For this review, take the finished solid that the model builds, in its own axes (mm). A direction names the side the tool comes from. Coordinates: 2 decimals unless noted, no trailing zeros. Write each loop counter-clockwise with the first axis right and the second up, starting at its lowest first coordinate (ties: lowest second). Pieces come first, ordered by that corner, then holes.
```python
from build123d import *

# Parameters (mm, degrees)
SKETCH_1_W      = 180
SKETCH_1_H      = 90
EXTRUDE_1_DEPTH = 3
FILLET_1_R      = 1
SKETCH_2_W      = 173
SKETCH_2_H      = 83
EXTRUDE_2_DEPTH = 3
SKETCH_5_R      = 2.695
SKETCH_5_R_2    = 0.895
SKETCH_5_R_3    = 2
SKETCH_5_R_4    = 0.7
SKETCH_5_R_5    = 3.225
SKETCH_5_R_6    = 1.425
EXTRUDE_3_DEPTH = 15.90000066


with BuildPart() as part:
    # 草图1 → 凸台-拉伸1 (new body)
    with BuildSketch(Plane(origin=(0, 0, 0), x_dir=(1, 0, 0), z_dir=(0, 1, 0))):
        Rectangle(SKETCH_1_W, SKETCH_1_H)
    extrude(amount=EXTRUDE_1_DEPTH)

    # 圆角1
    fillet_1_edges = [part.edges().sort_by_distance(p)[0] for p in [
        (0, 0, -45),
        (90, 0, 0),
        (0, 0, 45),
        (-90, 0, 0),
    ]]
    fillet(fillet_1_edges, radius=FILLET_1_R)

    # 草图2 → 凸台-拉伸2 (add)
    with BuildSketch(Plane(origin=(0, 3, 0), x_dir=(1, 0, 0), z_dir=(0, 1, 0))):
        Rectangle(SKETCH_2_W, SKETCH_2_H)
    extrude(amount=EXTRUDE_2_DEPTH)

    # 草图5 → 凸台-拉伸3 (add)
    # profile 1 of 5: a face of its own
    with BuildSketch(Plane(origin=(0, 3, 0), x_dir=(1, 0, 0), z_dir=(0, 1, 0))):
        with Locations((78.142, -4.005)):
            Circle(SKETCH_5_R)
        with Locations((78.142, -4.005)):
            Circle(SKETCH_5_R_2, mode=Mode.SUBTRACT)
    # profile 2 of 5: a face of its own
    with BuildSketch(Plane(origin=(0, 3, 0), x_dir=(1, 0, 0), z_dir=(0, 1, 0))):
        with Locations((83.5, -4.5)):
            Circle(SKETCH_5_R_3)
        with Locations((83.5, -4.5)):
            Circle(SKETCH_5_R_4, mode=Mode.SUBTRACT)
    # profile 3 of 5: a face of its own
    with BuildSketch(Plane(origin=(0, 3, 0), x_dir=(1, 0, 0), z_dir=(0, 1, 0))):
        with Locations((83.5, -38.5)):
            Circle(SKETCH_5_R_3)
        with Locations((83.5, -38.5)):
            Circle(SKETCH_5_R_4, mode=Mode.SUBTRACT)
    # profile 4 of 5: a face of its own
    with BuildSketch(Plane(origin=(0, 3, 0), x_dir=(1, 0, 0), z_dir=(0, 1, 0))):
        with Locations((14.882, -4.005)):
            Circle(SKETCH_5_R_5)
        with Locations((14.882, -4.005)):
            Circle(SKETCH_5_R_6, mode=Mode.SUBTRACT)
    # profile 5 of 5: a face of its own
    with BuildSketch(Plane(origin=(0, 3, 0), x_dir=(1, 0, 0), z_dir=(0, 1, 0))):
        with Locations((70.082, -39.015)):
            Circle(SKETCH_5_R_5)
        with Locations((70.082, -39.015)):
            Circle(SKETCH_5_R_6, mode=Mode.SUBTRACT)
    extrude(amount=EXTRUDE_3_DEPTH)


solid = part.part
```
1) Consider section A-A (y = 11.75). Count the separate pieces of the cut face and the enclosed holes in it, then the cut area to 3 significant figures.
2) Clearance check with flat-ended pins moving along their axes: P1, Ø3, axis at x = 48.5, z = 8, coming from the +Y side; P2, Ø1, axis at y = 5.5, z = 7.5, coming from the +X side; P3, Ø0.9, axis at x = 12.5, y = 4.5, coming from the -Z side; P4, Ø10, axis at x = -17, y = 14, coming from the -Z side. State where each tip first meets the part, or that it passes through.
3) Consider section C-C (x = -64.5). Give the boundary of the cut face in (y, z), then the cut area to 3 significant figures.
4) Consider section B-B (z = 23.5). Give the boundary of the cut face in (x, y).
5) The part is to be moulded in two halves that separate along X. For faces 3 (the face through (84.423, 12.36, 40.274)), 4 (the face through (16.3, 18.9, 4.7)), say which applies: pulls with the +X half, pulls with the -X half, needs draft (parallel to the pull), parting line crosses it, or undercut.
6) Tool access review of faces 1 (the face through (85.408, 12.36, 3.899)), 2 (the face through (79.3, 18.9, 4)): name each direction out of +Z, -Z, +X, -X, +Y, -Y from which nothing blocks a thin tool from reaching the whole face with its end or side.
7) For L1, parallel to Z at x = 83.5, y = 9; L2, parallel to X at y = 11, z = 38.5; L3, parallel to X at y = 4, z = 7, list the stretches that pass through material, from the lowest coordinate up.
Results:
1. separate pieces: 5
1. enclosed holes: 5
1. area: 94.9 mm2
2. P1: stops at y = 6
2. P2: stops at x = 86.5
2. P3: stops at z = -41.5
2. P4: passes through
3. outline: (0, -44) arc R1 ccw to (1, -45) - (3, -45) - (3, -41.5) - (6, -41.5) - (6, 41.5) - (3, 41.5) - (3, 45) - (1, 45) arc R1 ccw to (0, 44) - close
3. area: 519 mm2
4. outline: (-90, 1) arc R1 ccw to (-89, 0) - (89, 0) arc R1 ccw to (90, 1) - (90, 3) - (86.5, 3) - (86.5, 6) - (-86.5, 6) - (-86.5, 3) - (-90, 3) - close
5. face 3: undercut
5. face 4: needs draft
6. face 1: +Y
6. face 2: +Z, -Z, +X, -X, +Y
7. L1: z = 2.5 to 3.8, 5.2 to 6.5, 36.5 to 37.8, 39.2 to 40.5
7. L2: x = 66.9 to 68.75, 71.41 to 73.27, 81.5 to 82.8, 84.2 to 85.5
7. L3: x = -86.5 to 86.5
